The model under review builds one solid part; all positions refer to its coordinate system, in mm. Face numbers are marked on the shaded views. A direction names the side the tool comes from. Round coordinates to 2 decimals unless told otherwise and drop trailing zeros. Order: outer loops, then holes, each group sorted by start corner. A loop starts at its lowest first (then second) coordinate and runs counter-clockwise, first axis right, second up.
```python
from build123d import *

# Parameters (mm, degrees)
F1_DEPTH = 1.6


# Not quite as in the source:
# - a feature names something its author has since deleted; it is built from what else it names


with BuildPart() as f1:
    # F0 (on Top) → F1 (new body, symmetric)
    with BuildSketch(Plane.XY):
        with BuildLine():
            Line((-21, 3.2), (-21, 0))
            ThreePointArc((-21, 0), (0, -21), (21, 0))
            Line((21, 0), (19, 0))
            Line((19, 0), (19, 3.2))
            Line((19, 3.2), (11, 3.2))
            Line((11, 3.2), (11, 0))
            Line((11, 0), (3, 0))
            Line((3, 0), (3, 3.2))
            Line((3, 3.2), (-5, 3.2))
            Line((-5, 3.2), (-5, 0))
            Line((-5, 0), (-13, 0))
            Line((-13, 0), (-13, 3.2))
            Line((-13, 3.2), (-21, 3.2))
        make_face()
    extrude(amount=F1_DEPTH, both=True)


solid = f1.part
```
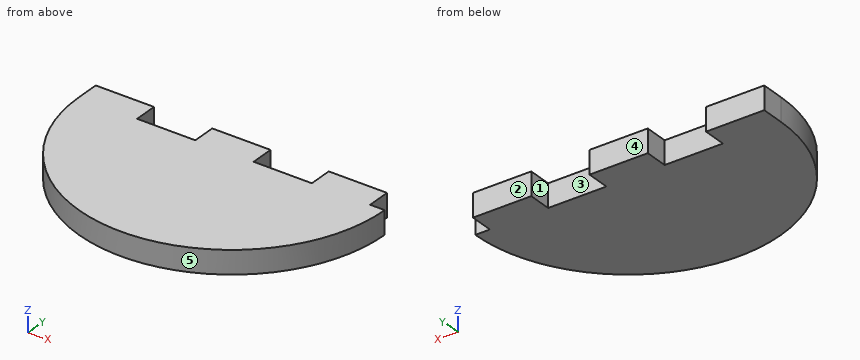
(1) To check wall thickness, follow probe 1 along X at (y, z) = (0.5, -0.6); probe 2 along Y at (x, z) = (0, -1.1); probe 3 along Y at (x, z) = (-13.5, 0.3). State the ranges of each line that lie inside material, in increasing order.
Data:
probe 1: x = -21 to -13, -5 to 3, 11 to 19
probe 2: y = -21 to 3.2
probe 3: y = -16.09 to 3.2
(2) Consider section B-B (x = -5.5). Write out the cut boundary in (y, z).
Data:
outline: (-20.27, -1.6) - (0, -1.6) - (0, 1.6) - (-20.27, 1.6) - close
(3) Insertion check: pin 1 (1.6 mm diameter, centred on x = 5, z = 0.5, fed in from +Y); pin 2 (1 mm diameter, centred on y = -18, z = 1.5, fed in from -X); pin 3 (1.6 mm diameter, centred on y = 2, z = 0, fed in from +X). Each pin has a flat end and moves straight along its axis. Give the tip position at first contact, or say it passes through.
Data:
pin 1: stops at y = 0
pin 2: stops at x = -11.61
pin 3: stops at x = 19
(4) Draft analysis for pull direction X (two halves, no side actions). For the marked faces 3, 4 and 5, state which applies: pulls with the +X half, pulls with the -X half, needs draft (parallel to the pull), parting line crosses it, or undercut.
Data:
face 3: undercut
face 4: needs draft
face 5: parting line crosses it
(5) For the marked faces 1 and 2, list the 3-axis set-ups (+Z, -Z, +X, -X, +Y, -Y) from which the entire face can be reached by the end or side of a thin tool; tool diameter is ignored.
Data:
face 1: +Z, -Z, +Y
face 2: +Z, -Z, +X, -X, +Y
(6) Consider section C-C (y = -15.5). Write out the cut boundary in (x, z), and give its area (3 significant figures).
Data:
outline: (-14.17, -1.6) - (14.17, -1.6) - (14.17, 1.6) - (-14.17, 1.6) - close
area: 90.7 mm2
(7) Consider section A-A (z = 1). Write out the cut boundary in (x, y), and give its area (3 significant figures).
Data:
outline: (-21, 0) arc R21 ccw to (21, 0) - (19, 0) - (19, 3.2) - (11, 3.2) - (11, 0) - (3, 0) - (3, 3.2) - (-5, 3.2) - (-5, 0) - (-13, 0) - (-13, 3.2) - (-21, 3.2) - close
area: 770 mm2
